```python
from build123d import *

# Parameters (mm, degrees)
SKETCH_1_W                  = 46
SKETCH_1_H                  = 43.413207239
EXTRUDE_1_DEPTH             = 41.6
SKETCH_2_W                  = 43
SKETCH_2_H                  = 40.1
CUT_EXTRUDE_1_DEPTH         = 64.417005312
SKETCH_3_W                  = 27
SKETCH_3_H                  = 10
CUT_EXTRUDE_2_DEPTH         = 78.334080456
SKETCH_4_W                  = 34.1
SKETCH_4_H                  = 33.413207239
CUT_EXTRUDE_3_DEPTH         = 86.49421033
SKETCH_5_W                  = 34.1
SKETCH_5_H                  = 33.413207239
CUT_EXTRUDE_4_DEPTH         = 87.284471372
CUT_EXTRUDE_5_DEPTH         = 78.334080456
HOLE_WIZARD_4_5_4_5_1_D     = 4.5
HOLE_WIZARD_4_5_4_5_1_DEPTH = 1.5
HOLE_WIZARD_4_5_4_5_2_D     = 4.5
HOLE_WIZARD_4_5_4_5_3_D     = 4.5
HOLE_WIZARD_4_5_4_5_3_DEPTH = 41.6
FILLET_1_R                  = 1
FILLET_2_R                  = 1.5
FILLET_3_R                  = 3
FILLET_4_R                  = 4
FILLET_5_R                  = 5.5
FILLET_6_R                  = 10


with BuildPart() as part:
    # 草图1 → 凸台-拉伸1 (new body)
    with BuildSketch(Plane(origin=(0, 0, -40.1), x_dir=(-1, 0, 0), z_dir=(0, 0, -1))):
        with Locations((0, -39.293396381)):
            Rectangle(SKETCH_1_W, SKETCH_1_H)
    extrude(amount=-EXTRUDE_1_DEPTH)

    # 草图2 → 切除-拉伸1 (cut, through all)
    with BuildSketch(Plane.XZ.offset(61)):
        with Locations((0, -20.05)):
            Rectangle(SKETCH_2_W, SKETCH_2_H)
    extrude(amount=-CUT_EXTRUDE_1_DEPTH, mode=Mode.SUBTRACT)

    # 草图3 → 切除-拉伸2 (cut, through all)
    with BuildSketch(Plane.XY.offset(1.5)):
        with Locations((0, -56)):
            Rectangle(SKETCH_3_W, SKETCH_3_H)
    extrude(amount=-CUT_EXTRUDE_2_DEPTH, mode=Mode.SUBTRACT)

    # 草图4 → 切除-拉伸3 (cut, through all)
    with BuildSketch(Plane(origin=(-21.5, 0, 0), x_dir=(0, 0, -1), z_dir=(1, 0, 0))):
        with Locations((23.05, -34.29339638)):
            Rectangle(SKETCH_4_W, SKETCH_4_H)
    extrude(amount=-CUT_EXTRUDE_3_DEPTH, mode=Mode.SUBTRACT)

    # 草图5 → 切除-拉伸4 (cut, through all)
    with BuildSketch(Plane(origin=(23, 0, 0), x_dir=(0, 0, -1), z_dir=(1, 0, 0))):
        with Locations((23.05, -34.29339638)):
            Rectangle(SKETCH_5_W, SKETCH_5_H)
    extrude(amount=-CUT_EXTRUDE_4_DEPTH, mode=Mode.SUBTRACT)

    # 草图6 → 切除-拉伸5 (cut, through all)
    with BuildSketch(Plane.XY.offset(1.5)):
        with BuildLine():
            Line((12.367486421, -17.586792761), (-12.367486421, -17.586792761))
            ThreePointArc((-12.367486421, -17.586792761), (0, -21.5), (12.367486421, -17.586792761))
        make_face()
    extrude(amount=-CUT_EXTRUDE_5_DEPTH, mode=Mode.SUBTRACT)

    # Ø4.5 (4.5) 直径孔1
    with Locations(Plane(origin=(-21.5, 0, 0), x_dir=(0, 0, -1), z_dir=(1, 0, 0))):
        with Locations((20.1, -56), (35.1, -56)):
            Hole(HOLE_WIZARD_4_5_4_5_1_D / 2, depth=HOLE_WIZARD_4_5_4_5_1_DEPTH)

    # Ø4.5 (4.5) 直径孔2 (through all)
    with Locations(Plane.ZY.offset(-21.5)):
        with Locations((-20.1, -56), (-35.1, -56)):
            Hole(HOLE_WIZARD_4_5_4_5_2_D / 2)

    # Ø4.5 (4.5) 直径孔3
    with Locations(Plane.XY.offset(1.5)):
        with Locations((-14, -45.5), (-14, -23.086792761), (14, -23.086792761), (14, -45.5)):
            Hole(HOLE_WIZARD_4_5_4_5_3_D / 2, depth=HOLE_WIZARD_4_5_4_5_3_DEPTH)

    # 圆角1
    fillet_1_edges = [part.edges().sort_by_distance(p)[0] for p in [
        (-22.25, -61, -40.1),
        (-13.5, -61, 0.75),
        (13.5, -61, 0.75),
        (22.25, -61, -40.1),
        (-22.25, -51, -40.1),
        (-22.25, -17.586792761, -6),
        (22.25, -51, -40.1),
        (22.25, -17.586792761, -6),
    ]]
    fillet(fillet_1_edges, radius=FILLET_1_R)

    # 圆角2
    fillet_2_edges = [part.edges().sort_by_distance(p)[0] for p in [
        (-21.5, -39.293396381, 0),
        (21.5, -39.293396381, 0),
    ]]
    fillet(fillet_2_edges, radius=FILLET_2_R)

    # 圆角3
    fillet_3_edges = [part.edges().sort_by_distance(p)[0] for p in [
        (-23, -39.293396381, 1.5),
        (23, -39.293396381, 1.5),
    ]]
    fillet(fillet_3_edges, radius=FILLET_3_R)

    # 圆角4
    fillet_4_edges = [part.edges().sort_by_distance(p)[0] for p in [
        (-13.5, -51, 0.75),
        (13.5, -51, 0.75),
    ]]
    fillet(fillet_4_edges, radius=FILLET_4_R)

    # 圆角5
    fillet_5_edges = [part.edges().sort_by_distance(p)[0] for p in [
        (12.367486421, -17.586792761, 0.75),
        (-12.367486421, -17.586792761, 0.75),
    ]]
    fillet(fillet_5_edges, radius=FILLET_5_R)

    # 圆角6
    fillet_6_edges = [part.edges().sort_by_distance(p)[0] for p in [
        (-22.25, -51, -6),
        (22.25, -51, -6),
    ]]
    fillet(fillet_6_edges, radius=FILLET_6_R)


solid = part.part
```
Check sheet for the modelled part. Datum: model origin and axes. Units: mm. A direction names the side the tool comes from. Round coordinates to 2 decimals unless told otherwise and drop trailing zeros. Order: outer loops, then holes, each group sorted by start corner. A loop starts at its lowest first (then second) coordinate and runs counter-clockwise, first axis right, second up.
1) Tool access check on faces 1 (the flat face through (22, -51, -27)), 2 (the cylindrical face through (21.07, -38.99, -0.45)), 3 (the flat face through (0, -51, 1)), 4 (the flat face through (20.2, -17.587, 0.2)). Record the directions out of +Z, -Z, +X, -X, +Y, -Y that give a thin tool (end or side, any length) a straight path to the whole face; none if there is none.
2) Section check A-A (y = -56). Give the number of separate pieces and of enclosed holes in the cut face, and give its area (3 significant figures).
3) Section check D-D (y = -45.5). Record the boundary of the cut face in (x, z).
4) Section check B-B (z = -35.1). Record the boundary of the cut face in (x, y).
5) Go/stop test with flat-tipped pins: pin 1 Ø1.2 at (y, z) = (-58.5, 0.5) entering from +X; pin 2 Ø1.2 at (x, y) = (22.5, -29) entering from -Z; pin 3 Ø8 at (x, y) = (-7, -49.5) entering from -Z. Record where each tip stops, or that it passes through.
6) Scan lines: line 1 (X direction, y = -25, z = -4); line 2 (Y direction, x = -22, z = -35); line 3 (Z direction, x = 1, y = -26). Record each from-to range of solid material in increasing order.
7) Mould release check, pull along Y, two halves, no side actions. Record for faces 5 (the cylindrical face through (12.359, -52.203, 0.74)), 6 (the flat face through (22, -56, -40.1)), 7 (the cylindrical face through (-15.04, -25.08, 0.74)), 8 (the cylindrical face through (14.29, -43.27, 0.74)): +Y half, -Y half, draft (parallel to the pull), parting line (faces both ways), or undercut.
8) Section check C-C (z = -8). Record the boundary of the cut face in (x, y).
Result:
1. face 1: -Z, +X, -X, +Y
1. face 2: -Z, +Y, -Y
1. face 3: +Z, -Z, -Y
1. face 4: +Z, -Z, +X, -X, +Y
2. separate pieces: 6
2. enclosed holes: 0
2. area: 119 mm2
3. outline: (-23, -7.07) - (-21.5, -7.07) - (-21.5, -1.5) arc R1.5 cw to (-20, 0) - (-16.25, 0) - (-16.25, 1.5) - (-20, 1.5) arc R3 ccw to (-23, -1.5) - close; (-11.75, 0) - (11.75, 0) - (11.75, 1.5) - (-11.75, 1.5) - close; (16.25, 0) - (20, 0) arc R1.5 cw to (21.5, -1.5) - (21.5, -7.07) - (23, -7.07) - (23, -1.5) arc R3 ccw to (20, 1.5) - (16.25, 1.5) - close
4. outline: (-23, -61) - (-21.5, -61) - (-21.5, -58.25) - (-23, -58.25) - close; (-23, -53.75) - (-21.5, -53.75) - (-21.5, -51) - (-23, -51) - close; (21.5, -61) - (23, -61) - (23, -58.25) - (21.5, -58.25) - close; (21.5, -53.75) - (23, -53.75) - (23, -51) - (21.5, -51) - close
5. pin 1: stops at x = 22.65
5. pin 2: stops at z = -6
5. pin 3: stops at z = 0
6. line 1: x = -23 to -21.5, 21.5 to 23
6. line 2: y = -61 to -58.25, -53.75 to -51
6. line 3: z = 0 to 1.5
7. face 5: -Y half
7. face 6: draft
7. face 7: undercut
7. face 8: undercut
8. outline: (-23, -61) - (-21.5, -61) - (-21.5, -47) - (-23, -47) - close; (21.5, -61) - (23, -61) - (23, -47) - (21.5, -47) - close
